Build history of the part. All positions in model axes, mm. Round coordinates to 2 decimals unless told otherwise and drop trailing zeros. Order: outer loops, then holes, each group sorted by start corner. A loop starts at its lowest first (then second) coordinate and runs counter-clockwise, first axis right, second up. Notation, with made-up numbers: M 73.5,83 L 115.5,83 A31 ccw 115.5,113 Z; hole C 77.25,3.25 d3. An arc over 180 degrees is marked long. Use CSV: the item, a comma, the result in double quotes.
from build123d import *

# Parameters (mm, degrees)
SKETCH_1_R          = 9.7
EXTRUDE_1_DEPTH     = 4
SKETCH_3_R          = 0.8
CUT_EXTRUDE_1_DEPTH = 10


with BuildPart() as part:
    # 草图1 → 凸台-拉伸1 (new body)
    with BuildSketch(Plane.XY):
        with BuildLine():
            Line((12.718684308, 6), (236.224480753, 6))
            ThreePointArc((236.224480753, 6), (265.02547605, 0), (236.224480753, -6))
            Line((236.224480753, -6), (12.718684308, -6))
            ThreePointArc((12.718684308, -6), (-14.062891969, 0), (12.718684308, 6))
        make_face()
        Circle(SKETCH_1_R, mode=Mode.SUBTRACT)
        with Locations((250, 0)):
            Circle(SKETCH_1_R, mode=Mode.SUBTRACT)
    extrude(amount=EXTRUDE_1_DEPTH)

    # 草图3 → 切除-拉伸1 (cut)
    with BuildSketch(Plane.XY.offset(4)):
        with Locations((9.7, 0)):
            Circle(SKETCH_3_R)
        with Locations((259.7, 0)):
            Circle(SKETCH_3_R)
    extrude(amount=-CUT_EXTRUDE_1_DEPTH, mode=Mode.SUBTRACT)


solid = part.part
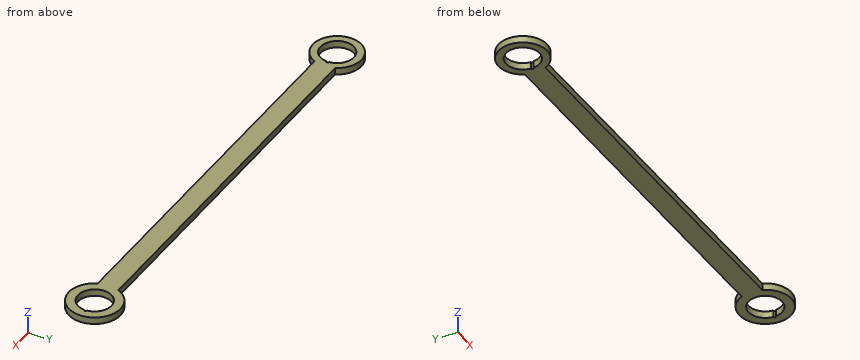
(1) Cut at A-A, the plane x = 250. Give the cut face in (y, z).
Answer block:
outline,"M -15.03,0 L -9.7,0 L -9.7,4 L -15.03,4 Z; M 9.7,0 L 15.03,0 L 15.03,4 L 9.7,4 Z"
(2) Drop flat-ended pins along their axis: pin 1 (1.5 mm diameter, centred on y = 1, z = 2, fed in from -X); pin 2 (1 mm diameter, centred on x = 210.5, z = 0.5, fed in from +Y); pin 3 (2 mm diameter, centred on x = 120.5, z = 2, fed in from -Y); pin 4 (1.5 mm diameter, centred on y = -0.5, z = 3, fed in from +X). Give the stop position or say it passes through.
Answer block:
pin 1,"stops at x = -14.06"
pin 2,"stops at y = 6"
pin 3,"stops at y = -6"
pin 4,"stops at x = 265.03"
(3) Wall check: line 1 (X direction, y = 0, z = 1.7); line 2 (Y direction, x = 0, z = 1.4); line 3 (Y direction, x = 250, z = 1.55). Give the ranges that are in metal, low to high. Write a range as from..to.
Answer block:
line 1,"x = -14.06..-9.7, 10.5..240.3, 260.5..265.03"
line 2,"y = -14.06..-9.7, 9.7..14.06"
line 3,"y = -15.03..-9.7, 9.7..15.03"
(4) Cut at B-B, the plane z = 2.9. Give the cut face in (x, y), and give its area (3 significant figures).
Answer block:
outline,"M 12.72,-6 L 236.22,-6 A15.03 ccw long 236.22,6 L 12.72,6 A14.06 ccw long Z; hole M 9.67,-0.8 A0.8 ccw long 9.67,0.8 A9.7 ccw long Z; hole M 259.67,-0.8 A0.8 ccw long 259.67,0.8 A9.7 ccw long Z"
area,"3,400 mm²"
(5) Cut at C-C, the plane x = 127.5. Give the cut face in (y, z).
Answer block:
outline,"M -6,0 L 6,0 L 6,4 L -6,4 Z"
